Could you check a few things on this model? Use its own coordinates, in mm. A direction names the side the tool comes from. Give positions to 0.01 mm unless a question says otherwise; leave off trailing zeros. Loops run counter-clockwise (first coordinate to the right, second up) from the corner with the lowest first, then second, coordinate; pieces in that order, holes last. Notation, with made-up numbers: (11, -18) - (43, -18) arc R33 cw to (43, 18) - close; hole circle Ø1 at (73, 49). An arc over 180 degrees is marked (long way). One line per item, written item: value. Start each with the question number.
Q1. For faces 4 (the face through (0, -34.925, 229)), 5 (the face through (0, 38.1, 229)), which set-ups out of +Z, -Z, +X, -X, +Y, -Y let a thin tool reach every point of the face, with its end or its side?
Q2. I want a section at B-B (y = 3.5). Please give me the cut outline in (x, z) (3 decimals).
Q3. If I drill on line 1 (Y direction, x = -6, z = 249) (3 decimals); line 2 (X direction, y = 14.5, z = 281) (3 decimals), over which ranges is the centre line in solid material (lowest first)? Write a range as from..to.
Q4. If we mould it in two halves opening along X, with no side actions, what happens to faces 1 (the face through (-10, 3, 0)), 2 (the face through (-12.7, -1, 229)), 3 (the face through (9.525, 0, 229))? For each: released by +X, released by -X, zero draft, split by the parting line, or undercut.
Q5. I'm going to push a flat-ended pin straight in: P1, Ø5.5, axis at y = -23.749, z = 403.225, coming from the -X side. Where does the tip first touch, or does it pass through?
Q6. I want a section at A-A (z = 302.5). Please give me the cut outline in (x, y) (3 decimals).
```python
from build123d import *

# Parameters (mm, degrees)
SKETCH1_W                   = 25.4
SKETCH1_H                   = 76.2
SKETCH1_W_2                 = 19.05
SKETCH1_H_2                 = 69.85
BOSS_EXTRUDE3_DEPTH         = 463.55
SKETCH6_R                   = 3.175
CUT_EXTRUDE1_DEPTH          = 806.45
F_1_4_0_25_DIAMETER_HOLE1_D = 6.35
F_1_4_0_25_DIAMETER_HOLE2_D = 6.35
F_1_4_0_25_DIAMETER_HOLE3_D = 6.35


with BuildPart() as part:
    # Sketch1 → Boss-Extrude3 (new body)
    with BuildSketch(Plane.XY):
        Rectangle(SKETCH1_W, SKETCH1_H)
        Rectangle(SKETCH1_W_2, SKETCH1_H_2, mode=Mode.SUBTRACT)
    extrude(amount=BOSS_EXTRUDE3_DEPTH)

    # Sketch6 → Cut-Extrude1 (cut)
    with BuildSketch(Plane(origin=(0, -38.1, 0), x_dir=(-1, 0, 0), z_dir=(0, -1, 0))):
        with Locations(Location((0, -9.525, 0), (0, 0, 180))):
            Circle(SKETCH6_R)
        with Locations(Location((0, -34.925, 0), (0, 0, 180))):
            Circle(SKETCH6_R)
        with Locations(Location((0, -454.025, 0), (0, 0, 180))):
            Circle(SKETCH6_R)
        with Locations(Location((0, -428.625, 0), (0, 0, 180))):
            Circle(SKETCH6_R)
    extrude(amount=-CUT_EXTRUDE1_DEPTH, mode=Mode.SUBTRACT)

    # 1/4 (0.25) Diameter Hole1 (through all)
    with Locations(Plane.ZY.offset(12.7)):
        with Locations((136.525, 27.051), (111.125, 27.051), (136.525, -23.749), (111.125, -23.749), (327.025, 27.051), (352.425, 27.051), (327.025, -23.749), (352.425, -23.749)):
            Hole(F_1_4_0_25_DIAMETER_HOLE1_D / 2)

    # 1/4 (0.25) Diameter Hole2 (through all)
    with Locations(Plane.ZY.offset(12.7)):
        with Locations((34.925, 27.051), (60.325, 27.051), (34.925, -23.749), (60.325, -23.749)):
            Hole(F_1_4_0_25_DIAMETER_HOLE2_D / 2)

    # 1/4 (0.25) Diameter Hole3 (through all)
    with Locations(Plane.ZY.offset(12.7)):
        with Locations((403.225, 27.051), (428.625, 27.051), (403.225, -23.749), (428.625, -23.749)):
            Hole(F_1_4_0_25_DIAMETER_HOLE3_D / 2)


solid = part.part
```
Worked answers:
1. face 4: +Z, -Z
1. face 5: +Z, -Z, +X, -X, +Y
2. outline: (-12.7, 0) - (-9.525, 0) - (-9.525, 463.55) - (-12.7, 463.55) - close; (9.525, 0) - (12.7, 0) - (12.7, 463.55) - (9.525, 463.55) - close
3. line 1: y = -38.1..-34.925, 34.925..38.1
3. line 2: x = -12.7..-9.525, 9.525..12.7
4. face 1: zero draft
4. face 2: released by -X
4. face 3: undercut
5. P1: passes through
6. outline: (-12.7, -38.1) - (12.7, -38.1) - (12.7, 38.1) - (-12.7, 38.1) - close; hole (-9.525, -34.925) - (9.525, -34.925) - (9.525, 34.925) - (-9.525, 34.925) - close
